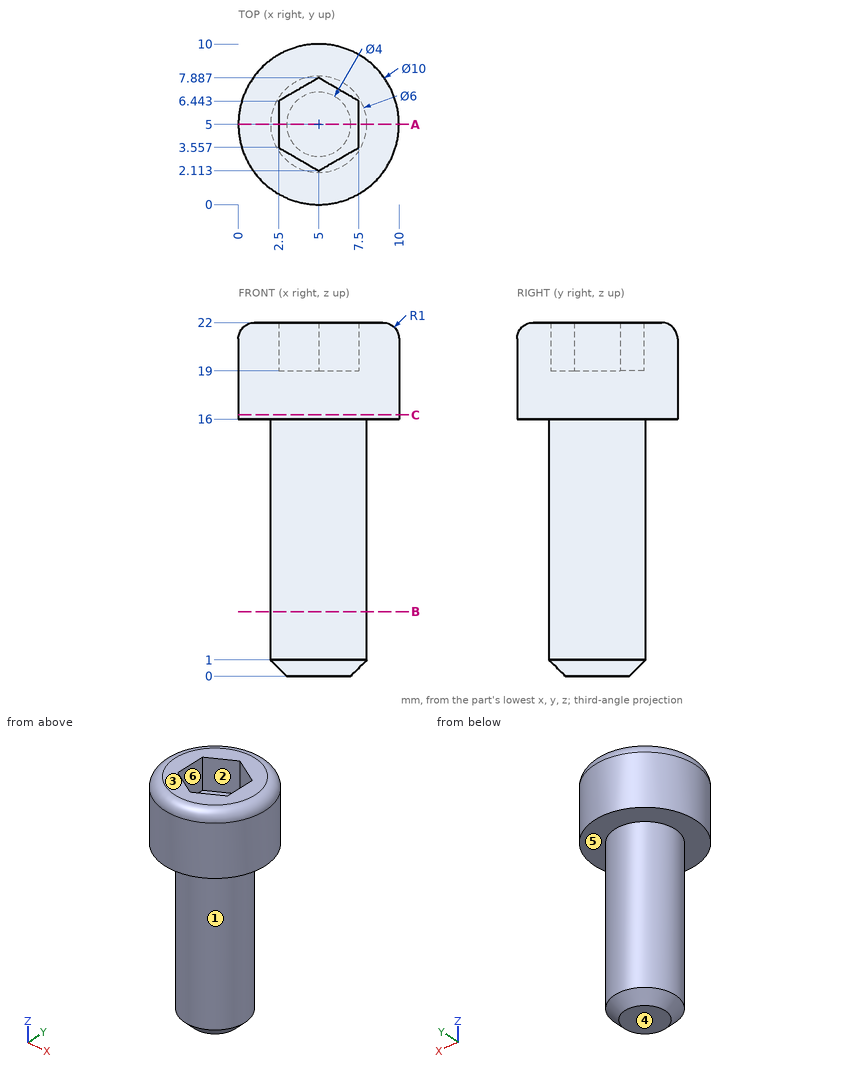
Check sheet for the drawn part. Datum: minimum x, y, z corner. Units: mm. A direction names the side the tool comes from. Round coordinates to 2 decimals unless told otherwise and drop trailing zeros. Order: outer loops, then holes, each group sorted by start corner. A loop starts at its lowest first (then second) coordinate and runs counter-clockwise, first axis right, second up.
(1) Access from +Z, -Z, +X, -X, +Y, -Y to the whole of each face (thin tool, end or side, straight path). Record for the marked faces 4, 5 and 6.
(2) Cross-section at C-C, the plane z = 16.25. Enter the section's corners in (x, y).
(3) Draft check along X on the marked faces 1, 2 and 3. Enter one of: pulls with the +X half, pulls with the -X half, needs draft (parallel to the pull), parting line crosses it, or undercut.
(4) Scan lines: probe 1 along Z at (x, y) = (4.5, 3.75); probe 2 along Z at (x, y) = (1.5, 5.5); probe 3 along X at (y, z) = (7.75, 15) (1 decimal). Record each from-to range of solid material in increasing order.
(5) Cross-section at A-A, the plane y = 5. Enter the section's corners in (x, z).
(6) Cross-section at B-B, the plane z = 4. Enter the section's corners in (x, y).
(7) Go/stop test with flat-tipped pins: P1, Ø5, axis at x = 8.5, z = 17.5, coming from the +Y side; P2, Ø2, axis at x = 3.5, z = 16.5, coming from the -Y side (1 decimal); P3, Ø1, axis at y = 6, z = 10, coming from the -X side. Record where each tip stops, or that it passes through.
Check sheet entries:
1. face 4: -Z, +X, -X, +Y, -Y
1. face 5: -Z
1. face 6: +Z
2. outline: circle Ø10 at (5, 5)
3. face 1: parting line crosses it
3. face 2: undercut
3. face 3: needs draft
4. probe 1: z = 0 to 19
4. probe 2: z = 16 to 22
4. probe 3: x = 3.8 to 6.2
5. outline: (0, 16) - (2, 16) - (2, 1) - (3, 0) - (7, 0) - (8, 1) - (8, 16) - (10, 16) - (10, 21) arc R1 ccw to (9, 22) - (7.5, 22) - (7.5, 19) - (2.5, 19) - (2.5, 22) - (1, 22) arc R1 ccw to (0, 21) - close
6. outline: circle Ø6 at (5, 5)
7. P1: stops at y = 9.9
7. P2: stops at y = 0
7. P3: stops at x = 2.04
